Could you check a few things on this model? Use its own coordinates, in mm. A direction names the side the tool comes from. Give positions to 0.01 mm unless a question says otherwise; leave off trailing zeros. Loops run counter-clockwise (first coordinate to the right, second up) from the corner with the lowest first, then second, coordinate; pieces in that order, holes last.
1. For P1, Ø5, axis at x = 5.5, y = -11.5, coming from the -Z side; P2, Ø2, axis at x = 2, y = -9, coming from the -Z side; P3, Ø0.9, axis at x = -7, z = 3.5, coming from the -Y side, each with a flat end and sliding along its axis, tell me the tip position at first contact or that it passes through.
2. Imagine slicing it at B-B (y = -14.75). List the corners of the cut face in (x, z) for me, plus the area to 3 significant figures.
3. Imagine slicing it at D-D (y = -17.25). List the corners of the cut face in (x, z) for me.
4. Imagine slicing it at A-A (z = 2.75). List the corners of the cut face in (x, y) for me.
5. Thinking about a two-plate mould opening in Y: for faces 1 (the flat face through (6.275, -6, 5)), 2 (the flat face through (8.643, -9.649, 2.958)), 3 (the flat face through (-2, -11, 10)), which applies, +Y half, -Y half, draft (parallel to the pull), parting line (faces both ways), or undercut?
6. I need wall thicknesses on line 1 along X through (y, z) = (-6.25, 2.5); line 2 along Y through (x, z) = (8.75, 9.5); line 3 along Y through (x, z) = (-7.5, 0.5). Which ranges of each line are inside material? Lowest first, please.
7. For faces 4 (the cylindrical face through (-5.594, -21.431, 9.43)), 5 (the cylindrical face through (9.9, -7.583, 10.165)), 6 (the cylindrical face through (7.026, -5.726, 9.521)), 7 (the flat face through (-6.09, -21.21, 9.59)), which set-ups out of +Z, -Z, +X, -X, +Y, -Y let a thin tool reach every point of the face, with its end or its side?
8. Imagine slicing it at C-C (z = 7). List the corners of the cut face in (x, y) for me, plus the area to 3 significant figures.
```python
from build123d import *

# Parameters (mm, degrees)
BOSS_EXTRUDE1_DEPTH      = 11
BOSS_EXTRUDE2_START      = 11
BOSS_EXTRUDE2_DEPTH      = 1
SKETCH6_W                = 12
SKETCH6_H                = 1
UPPER_TUBE_OPENING_DEPTH = 10
LOWER_TUBE_OPENING_DEPTH = 1
SKETCH4_R                = 0.800000001
SKETCH4_R_2              = 0.800000002
SCREW_HOLES_DEPTH        = 29.262100116
SCREW_START              = 11
SKETCH5_R                = 1.25
SCREW_HEADS_DEPTH        = 3
FILLET1_R                = 2
CUT_EXTRUDE1_DEPTH       = 6


with BuildPart() as part:
    # Sketch2 → Boss-Extrude1 (new body)
    with BuildSketch(Plane.XY):
        Polygon((-6.378060684, -22.912224964), (3.521434253, -13.012730028), (8.11762833, -17.608924106), (12.360269017, -13.366283419), (10.274522062, -11.280536464), (10.274522062, -3.780536464), (-9.725477938, -3.780536464), (-9.725477938, -19.56480771), align=None)
        Polygon((-5.725477938, -7.780536464), (-5.725477938, -4.780536464), (6.274522063, -4.780536464), (6.274522063, -8.845428655), (-6.378060684, -21.498011402), (-8.725477938, -19.150594148), (-8.725477938, -7.780536464), align=None, mode=Mode.SUBTRACT)
    extrude(amount=BOSS_EXTRUDE1_DEPTH)

    # Sketch3 → Boss-Extrude2 (add)
    with BuildSketch(Plane.XY.offset(BOSS_EXTRUDE2_START)):
        Polygon((-6.378060684, -22.912224964), (3.521434253, -13.012730028), (8.11762833, -17.608924106), (12.360269017, -13.366283419), (10.274522062, -11.280536464), (10.274522062, -3.780536464), (-9.725477938, -3.780536464), (-9.725477938, -19.56480771), align=None)
    extrude(amount=-BOSS_EXTRUDE2_DEPTH)

    # Sketch6 → Upper Tube Opening (cut)
    with BuildSketch(Plane.XY):
        with Locations((0.274522062, -4.280536464)):
            Rectangle(SKETCH6_W, SKETCH6_H)
    extrude(amount=UPPER_TUBE_OPENING_DEPTH, mode=Mode.SUBTRACT)

    # Sketch7 → Lower Tube Opening (cut)
    with BuildSketch(Plane(origin=(8.26708214, -8.26708214, 0), x_dir=(0, 0, -1), z_dir=(0.7071067811865477, -0.7071067811865475, 0))):
        with BuildLine():
            Line((-8, -19.711359605), (0, -19.711359605))
            Line((0, -19.711359605), (0, -6.711359605))
            Line((0, -6.711359605), (-10, -6.711359605))
            Line((-10, -6.711359605), (-10, -17.711359605))
            ThreePointArc((-10, -17.711359605), (-9.414213562, -19.125573167), (-8, -19.711359605))
        make_face()
    extrude(amount=-LOWER_TUBE_OPENING_DEPTH, mode=Mode.SUBTRACT)

    # Sketch4 → Screw Holes (cut, through all)
    with BuildSketch(Plane.XY):
        with Locations((9.178288502, -14.426943591)):
            Circle(SKETCH4_R)
        with Locations((7.056968158, -12.305623247)):
            Circle(SKETCH4_R)
        with Locations((-7.725477938, -5.780536464)):
            Circle(SKETCH4_R_2)
        with Locations((8.274522062, -5.780536464)):
            Circle(SKETCH4_R_2)
    extrude(amount=SCREW_HOLES_DEPTH, mode=Mode.SUBTRACT)

    # Sketch5 → Screw Heads (cut)
    with BuildSketch(Plane.XY.offset(SCREW_START)):
        with Locations((-7.725477938, -5.780536464)):
            Circle(SKETCH5_R)
        with Locations((8.274522062, -5.780536464)):
            Circle(SKETCH5_R)
        with Locations((7.056968158, -12.305623247)):
            Circle(SKETCH5_R)
        with Locations((9.178288502, -14.426943591)):
            Circle(SKETCH5_R)
    extrude(amount=-SCREW_HEADS_DEPTH, mode=Mode.SUBTRACT)

    # Fillet1
    # the kernel refuses this fillet: 2 mm, written as the material it takes off along each edge
    with BuildSketch(Plane(origin=(10.274522062, -16.280536464, 11), x_dir=(-1, 0, 0), z_dir=(0, 1, 0))) as fillet1_piece_1_section:
        with BuildLine():
            CenterArc((FILLET1_R, -FILLET1_R), FILLET1_R, 90, 90)
            Line((0, -FILLET1_R), (0, 0))
            Line((0, 0), (FILLET1_R, 0))
        make_face()
    fillet1_piece_1 = extrude(amount=17.5, mode=Mode.PRIVATE)
    fillet1_piece_1 = split(fillet1_piece_1, bisect_by=Plane(origin=(6.821503017, -7.82751742, 10.5380934), z_dir=(0.707106781186547, 0.7071067811865481, 0)), keep=Keep.TOP, mode=Mode.PRIVATE)
    add(fillet1_piece_1, mode=Mode.SUBTRACT)
    with BuildSketch(Plane(origin=(-9.725477938, 1.219463536, 11), x_dir=(1, 0, 0), z_dir=(0, -1, 0))) as fillet1_piece_2:
        with BuildLine():
            CenterArc((FILLET1_R, -FILLET1_R), FILLET1_R, 90, 90)
            Line((0, -FILLET1_R), (0, 0))
            Line((0, 0), (FILLET1_R, 0))
        make_face()
    extrude(amount=25.784271246, mode=Mode.SUBTRACT)
    with BuildSketch(Plane(origin=(-13.261011844, -16.029273804, 11), x_dir=(0.7071067811865474, 0.7071067811865478, 0), z_dir=(0.7071067811865478, -0.7071067811865474, 0))) as fillet1_piece_3:
        with BuildLine():
            CenterArc((FILLET1_R, -FILLET1_R), FILLET1_R, 90, 90)
            Line((0, -FILLET1_R), (0, 0))
            Line((0, 0), (FILLET1_R, 0))
        make_face()
    extrude(amount=14.73396288, mode=Mode.SUBTRACT)

    # Sketch10 → Cut-Extrude1 (cut)
    with BuildSketch(Plane.XY):
        Polygon((12.360269017, -13.366283419), (8.11762833, -17.608924106), (2.814327472, -12.305623247), (7.056968158, -8.06298256), align=None)
    extrude(amount=CUT_EXTRUDE1_DEPTH, mode=Mode.SUBTRACT)


solid = part.part
```
Derived:
1. P1: stops at z = 6
1. P2: stops at z = 10
1. P3: stops at y = -22.74
2. outline: (-9.73, 0) - (-8.73, 0) - (-8.73, 10) - (1.78, 10) - (1.78, 11) - (-7.73, 11) arc R2 ccw to (-9.73, 9) - close; (5.26, 6) - (8.45, 6) - (8.45, 8) - (7.97, 8) - (7.97, 11) - (5.26, 11) - close; (9.91, 6) - (10.98, 6) - (10.98, 11) - (10.39, 11) - (10.39, 8) - (9.91, 8) - close
2. area: 39.1 mm2
3. outline: (-9.73, 0) - (-8.73, 0) - (-8.73, 10) - (-0.72, 10) - (-0.72, 11) - (-7.73, 11) arc R2 ccw to (-9.73, 9) - close; (7.76, 6) - (8.48, 6) - (8.48, 11) - (7.76, 11) - close
4. outline: (-9.73, -19.56) - (-6.38, -22.91) - (-5.67, -22.21) - (-8.73, -19.15) - (-8.73, -7.78) - (-5.73, -7.78) - (-5.73, -3.78) - (-9.73, -3.78) - close; (6.27, -8.85) - (7.06, -8.06) - (10.27, -11.28) - (10.27, -3.78) - (6.27, -3.78) - close; hole circle Ø1.6 at (-7.73, -5.78); hole circle Ø1.6 at (8.27, -5.78)
5. face 1: draft
5. face 2: -Y half
5. face 3: undercut
6. line 1: x = -9.73 to -8.37, -7.08 to -5.73, 6.27 to 7.63, 8.92 to 10.27
6. line 2: y = -16.98 to -15.6, -13.25 to -6.94, -4.62 to -3.78
6. line 3: y = -21.79 to -20.38, -7.78 to -6.55, -5.01 to -3.78
7. face 4: -Z, +X
7. face 5: +Z, +X, +Y
7. face 6: +Z
7. face 7: -Z
8. outline: (-9.73, -19.56) - (-6.38, -22.91) - (-5.67, -22.21) - (-8.73, -19.15) - (-8.73, -7.78) - (-5.73, -7.78) - (-5.73, -3.78) - (-9.73, -3.78) - close; (2.81, -12.31) - (8.12, -17.61) - (12.36, -13.37) - (10.27, -11.28) - (10.27, -3.78) - (6.27, -3.78) - (6.27, -8.85) - close; hole circle Ø1.6 at (-7.73, -5.78); hole circle Ø1.6 at (7.06, -12.31); hole circle Ø1.6 at (8.27, -5.78); hole circle Ø1.6 at (9.18, -14.43)
8. area: 91.7 mm2
